The figure shows three views and two pictorial views of one solid part (mm, origin at its lowest corner). Answer the questions. Coordinates: 2 decimals unless noted, no trailing zeros. Loops run counter-clockwise (first coordinate to the right, second up) from the corner with the lowest first, then second, coordinate; pieces in that order, holes last. Notation, with made-up numbers: M -26,54.25 L 31,54.25 A16 ccw 31,61.25 Z; hole C -18.5,60.5 d7. An arc over 180 degrees is marked long. Return JSON: item names as keys, results as strings. Group by question number.
1. Straight lines are drawn through the part: L1, parallel to Y at x = 25, z = 13.75; L2, parallel to Y at x = 25, z = 8; L3, parallel to Y at x = 36, z = 2.5. For each, find the intervals that lie inside material, in ascending order. Write a range as from..to.
2. Given P1, Ø6, axis at x = 11.5, z = 16, coming from the -Y side, flat-ended and moving along its own axis, determine where the tip first touches the part or whether it passes through.
3. Section D-D (x = 7.5) is taken. Write down the section's boundary in (y, z).
4. The mould has two halves that part along X. Classify the marked faces 1, 2 and 3: pulls with the +X half, pulls with the -X half, needs draft (parallel to the pull), parting line crosses it, or undercut.
5. Section B-B (x = 25) is taken. Write down the section's boundary in (y, z), then the cut area to 3 significant figures.
6. Section C-C (z = 13.5) is taken. Write down the section's boundary in (x, y), then the cut area to 3 significant figures.
7. Section A-A (y = 23) is taken. Write down the section's boundary in (x, z).
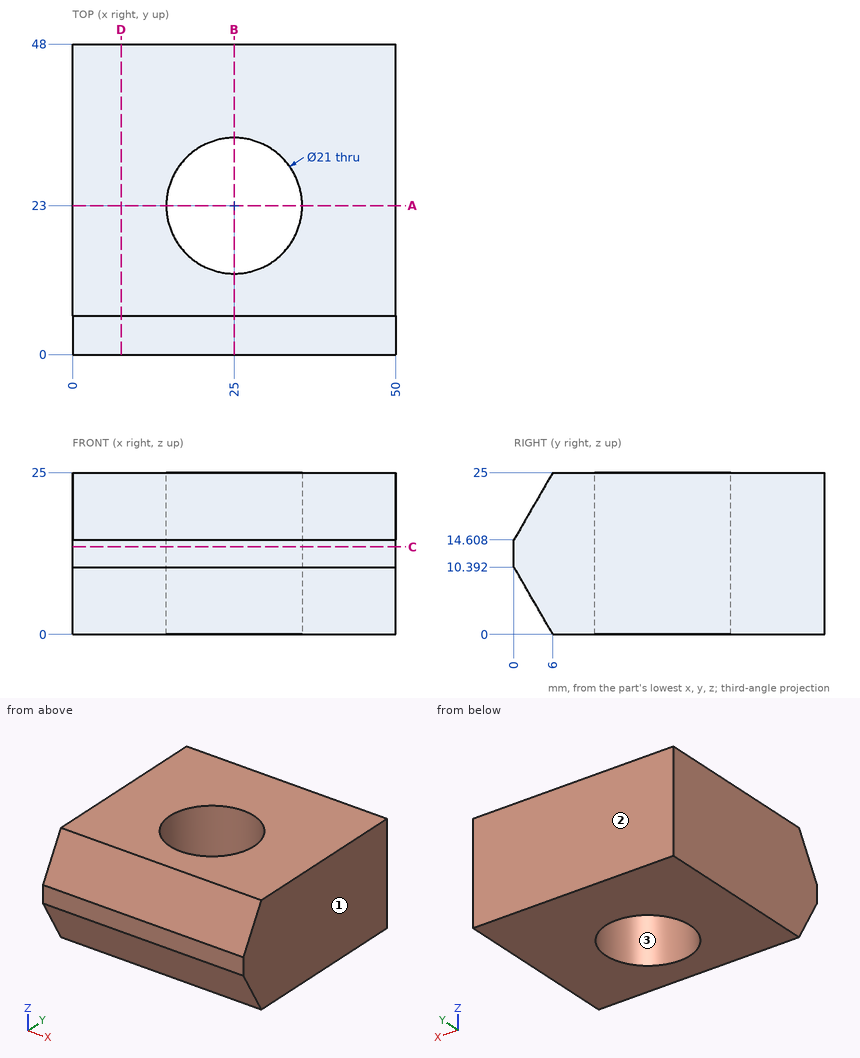
Worked out:
{
 "1": {"L1": "0..12.5, 33.5..48", "L2": "1.38..12.5, 33.5..48", "L3": "4.56..48"},
 "2": {"P1": "y = 0"},
 "3": {"outline": "M 0,10.39 L 6,0 L 48,0 L 48,25 L 6,25 L 0,14.61 Z"},
 "4": {"face 1": "pulls with the +X half", "face 2": "needs draft", "face 3": "undercut"},
 "5": {"outline": "M 0,10.39 L 6,0 L 12.5,0 L 12.5,25 L 6,25 L 0,14.61 Z; M 33.5,0 L 48,0 L 48,25 L 33.5,25 Z", "area": "613 mm^2"},
 "6": {"outline": "M 0,0 L 50,0 L 50,48 L 0,48 Z; hole C 25,23 d21", "area": "2,050 mm^2"},
 "7": {"outline": "M 0,0 L 14.5,0 L 14.5,25 L 0,25 Z; M 35.5,0 L 50,0 L 50,25 L 35.5,25 Z"}
}
